```python
from build123d import *

# Parameters (mm, degrees)
F3_DEPTH        = 2
F3_COPIES_COUNT = 8
F4_W            = 13
F4_H            = 2


# Not quite as in the source:
# - a pattern or mirror of a feature is missing from the dataset's text; its kind, count and spacing are read off the source's solid


with BuildPart() as f1:
    # F0 (on Right) → F1 (revolve)
    with BuildSketch(Plane.YZ):
        Polygon((0, 12), (0, 8), (19.8, 8), (19.8, 15), (22.3, 15), (27.8, 32.7), (29, 32.7), (29, 35), (25, 35), (16.5, 15), (10, 12.5), align=None)
    revolve(axis=Axis((0, 14.5, 0), (0, 1, 0)))

    # F2 (on Right) → F3 (join, symmetric)
    with BuildSketch(Plane.YZ):
        Polygon((27, 35), (25, 35), (17, 35), (12, 21), (17.5625, 17.5), (19.5625, 17.5), align=None)
    f3 = extrude(amount=F3_DEPTH, both=True)

    # F3_copies: F3 ×8 about axis
    f3_copies_axis = Axis((0, 0, 0), (0, 1, 0))
    for i in range(1, F3_COPIES_COUNT):
        add(f3.rotate(f3_copies_axis, i * 360 / F3_COPIES_COUNT))

    # F4 (on Right) → F5 (revolve, cut)
    with BuildSketch(Plane.YZ):
        with Locations((22.5, 36)):
            Rectangle(F4_W, F4_H)
    revolve(axis=Axis((0, 14.5, 0), (0, 1, 0)), mode=Mode.SUBTRACT)


solid = f1.part
```
Verification items for the finished model (mm, model axes). A direction names the side the tool comes from. Coordinates: 2 decimals unless noted, no trailing zeros. Loops run counter-clockwise (first coordinate to the right, second up) from the corner with the lowest first, then second, coordinate; pieces in that order, holes last. Notation, with made-up numbers: (86.25, 3) - (118.25, 3) arc R18 cw to (118.25, 8) - close; hole circle Ø6 at (18.5, -32). An arc over 180 degrees is marked (long way). Put each result on its own line as item: value.
Item 1: Section check C-C (y = 11). Enter the section's corners in (x, z).
Conclusion:
outline: circle Ø25.77 at (0, 0); hole circle Ø16 at (0, 0)
Item 2: Scan lines: line 1 along X through (y, z) = (28.25, 0); line 2 along Z through (x, y) = (-28, 17.5); line 3 along X through (y, z) = (21.6, 0). Record each from-to range of solid material in increasing order.
Conclusion:
line 1: x = -35 to -32.7, 32.7 to 35
line 2: z = -2 to 2
line 3: x = -35 to -15, 15 to 35
Item 3: Draft check along Z on faces 5 (the face through (-28, 18, -2)), 6 (the face through (-19.888, 14.535, -19.848)), 7 (the face through (1.539, 25.745, -34.966)). Enter one of: pulls with the +Z half, pulls with the -Z half, needs draft (parallel to the pull), parting line crosses it, or undercut.
Conclusion:
face 5: undercut
face 6: pulls with the -Z half
face 7: parting line crosses it
Item 4: Section check B-B (y = 6.5). Enter the section's corners in (x, z) (3 decimals), then the cut area to 3 significant figures.
Conclusion:
outline: circle Ø24.65 at (0, 0); hole circle Ø16 at (0, 0)
area: 276 mm2
Item 5: Gauge pin test, flat ends, axial feed: pin 1 Ø4 at (y, z) = (20, -25.5) entering from +X; pin 2 Ø6 at (x, z) = (-20, -10.5) entering from -Y; pin 3 Ø4 at (y, z) = (16.5, 26) entering from -X. Record the tip position at first contact, or that the pin passes through.
Conclusion:
pin 1: stops at x = 25.94
pin 2: stops at y = 18.45
pin 3: stops at x = -25.42
Item 6: Set-up check for faces 1 (the face through (18.58, 18.41, 21.41)), 2 (the face through (-21.41, 18.41, 18.58)), 3 (the face through (0.66, 21.068, -14.985)), 4 (the face through (28, 18, -2)): record each of +Z, -Z, +X, -X, +Y, -Y from which the full face is reachable in a straight line by a thin tool's end or side.
Conclusion:
face 1: +Z, -Y
face 2: -X, -Y
face 3: +Y
face 4: +X, -Y
